CAD build for the part. Positions are in the model's coordinates, mm. A direction names the side the tool comes from. Give positions to 0.01 mm unless a question says otherwise; leave off trailing zeros. Write each loop counter-clockwise with the first axis right and the second up, starting at its lowest first coordinate (ties: lowest second). Pieces come first, ordered by that corner, then holes. Notation, with made-up numbers: (31.25, -14) -> (88.25, -14) arc R18 ccw to (88.25, 15) -> close; hole circle Ø4 at (83, -26.75). An arc over 180 degrees is marked (long way). Answer in a Markdown table with one row per item. Add a question column.
```python
from build123d import *

# Parameters (mm, degrees)
SKETCH3_W           = 800
SKETCH3_H           = 170
SKETCH3_W_2         = 740
SKETCH3_H_2         = 150
BOSS_EXTRUDE1_DEPTH = 10
BOSS_EXTRUDE2_DEPTH = 500
SKETCH5_W           = 800
SKETCH5_H           = 170
SKETCH5_W_2         = 740
SKETCH5_H_2         = 148.57875962
BOSS_EXTRUDE3_DEPTH = 10
SKETCH7_R           = 74.28937981
BOSS_EXTRUDE6_DEPTH = 500
SKETCH6_R           = 10
CUT_EXTRUDE1_DEPTH  = 521
BOSS_EXTRUDE8_DEPTH = 50
CUT_EXTRUDE2_DEPTH  = 20
SKETCH10_W          = 10.613943808
SKETCH10_H          = 30
BOSS_EXTRUDE9_DEPTH = 530


with BuildPart() as part:
    # Sketch3 → Boss-Extrude1 (new body)
    with BuildSketch(Plane.XY):
        with Locations((140, 0)):
            Rectangle(SKETCH3_W, SKETCH3_H)
        with Locations((140, 0)):
            Rectangle(SKETCH3_W_2, SKETCH3_H_2, mode=Mode.SUBTRACT)
    extrude(amount=BOSS_EXTRUDE1_DEPTH)

    # Sketch4 → Boss-Extrude2 (add)
    with BuildSketch(Plane.XY.offset(10)):
        with BuildLine():
            Line((-245, 84.28937981), (525, 84.28937981))
            ThreePointArc((525, 84.28937981), (609.28937981, 0), (525, -84.28937981))
            Line((525, -84.28937981), (-245, -84.28937981))
            ThreePointArc((-245, -84.28937981), (-329.28937981, 0), (-245, 84.28937981))
        make_face()
        with BuildLine():
            Line((-245, 74.28937981), (525, 74.28937981))
            ThreePointArc((525, 74.28937981), (599.28937981, 0), (525, -74.28937981))
            Line((525, -74.28937981), (-245, -74.28937981))
            ThreePointArc((-245, -74.28937981), (-319.28937981, 0), (-245, 74.28937981))
        make_face(mode=Mode.SUBTRACT)
    extrude(amount=BOSS_EXTRUDE2_DEPTH)

    # Sketch5 → Boss-Extrude3 (add)
    with BuildSketch(Plane.XY.offset(510)):
        with Locations((140, 0)):
            Rectangle(SKETCH5_W, SKETCH5_H)
        with Locations((140, 0)):
            Rectangle(SKETCH5_W_2, SKETCH5_H_2, mode=Mode.SUBTRACT)
    extrude(amount=BOSS_EXTRUDE3_DEPTH)

    # Sketch7 → Boss-Extrude6 (add)
    with BuildSketch(Plane.XY.offset(10)):
        with Locations((-245, 0)):
            Circle(SKETCH7_R)
        with Locations((525, 0)):
            Circle(SKETCH7_R)
    extrude(amount=BOSS_EXTRUDE6_DEPTH)

    # Sketch6 → Cut-Extrude1 (cut, through all)
    with BuildSketch(Plane.XY.offset(520)):
        with Locations((-245, 0)):
            Circle(SKETCH6_R)
        with Locations((525, 0)):
            Circle(SKETCH6_R)
    extrude(amount=-CUT_EXTRUDE1_DEPTH, mode=Mode.SUBTRACT)

    # Sketch8 → Boss-Extrude8 (add)
    with BuildSketch(Plane.XY.offset(520)):
        with BuildLine():
            Line((-245, 200), (525, 200))
            ThreePointArc((525, 200), (725, 0), (525, -200))
            Line((525, -200), (-245, -200))
            ThreePointArc((-245, -200), (-445, 0), (-245, 200))
        make_face()
    boss_extrude8 = extrude(amount=BOSS_EXTRUDE8_DEPTH)

    # Sketch9 → Cut-Extrude2 (cut)
    with BuildSketch(Plane(origin=(0, 0, 520), x_dir=(-1, 0, 0), z_dir=(0, 0, -1))):
        with BuildLine():
            Line((-525, 172.743663041), (245, 172.743663041))
            ThreePointArc((245, 172.743663041), (417.743663041, 0), (245, -172.743663041))
            Line((245, -172.743663041), (-525, -172.743663041))
            ThreePointArc((-525, -172.743663041), (-697.743663041, 0), (-525, 172.743663041))
        make_face()
        with BuildLine():
            Line((-525, -142.743663041), (245, -142.743663041))
            ThreePointArc((245, -142.743663041), (387.743663041, 0), (245, 142.743663041))
            Line((245, 142.743663041), (-525, 142.743663041))
            ThreePointArc((-525, 142.743663041), (-667.743663041, 0), (-525, -142.743663041))
        make_face(mode=Mode.SUBTRACT)
    cut_extrude2 = extrude(amount=-CUT_EXTRUDE2_DEPTH, mode=Mode.SUBTRACT)

    # Sketch10 → Boss-Extrude9 (add)
    with BuildSketch(Plane(origin=(0, 0, 540), x_dir=(-1, 0, 0), z_dir=(0, 0, -1))):
        with Locations((135.520291363, 157.743663041)):
            Rectangle(SKETCH10_W, SKETCH10_H)
        with Locations((-164.479708637, 157.743663041)):
            Rectangle(SKETCH10_W, SKETCH10_H)
        with Locations((-464.479708637, 157.743663041)):
            Rectangle(SKETCH10_W, SKETCH10_H)
    extrude(amount=BOSS_EXTRUDE9_DEPTH)

    # Mirror1: Boss-Extrude8, Cut-Extrude2 across plane
    add(boss_extrude8.mirror(Plane(origin=(0, 0, 260), x_dir=(1, 0, 0), z_dir=(0, 0, -1))))
    add(cut_extrude2.mirror(Plane(origin=(0, 0, 260), x_dir=(1, 0, 0), z_dir=(0, 0, -1))), mode=Mode.SUBTRACT)


solid = part.part
```
Item 1: Slice it at C-C, the plane y = 159. List the corners of the cut face in (x, z), then the cut area to 3 significant figures.
Item 2: Probe L1, parallel to Z at x = 508.5, y = 4.5; L2, parallel to Y at x = 10.5, z = 169; L3, parallel to Z at x = -192.5, y = 62. List the from-to ranges inside material, lowest first. Write a range as from..to.
Item 3: Which spindle directions (+Z, -Z, +X, -X, +Y, -Y) get a long thin tool onto all of the face, cutting with end or side? Do faces 1 (the face through (145, -84.289, 256)), 2 (the face through (-417.7, 3.8, 529.9)), 3 (the face through (567, 1, 510)). Say none if no direction does.
Item 4: Slice it at A-A, the plane z = 403. List the corners of the cut face in (x, y).
Item 5: Mould opens along X. For faces 4 (the face through (609.27, 1.85, 256.5)), 5 (the face through (487, 1, 10)), 6 (the face through (-286, 1, 10)), 7 (the face through (487, 1, 510)) say: released by +X, released by -X, zero draft, split by the parting line, or undercut.
Item 6: Slice it at B-B, the plane x = 571.5. List the corners of the cut face in (y, z).
Item 7: Drop flat-ended pins along their axis: pin 1 Ø2 at (x, z) = (158, 200) entering from +Y; pin 2 Ø3 at (y, z) = (6.5, 514.5) entering from +X; pin 3 Ø3 at (x, z) = (-286.5, 136.5) entering from +Y. Give the stop position or say it passes through.
Answer key:
| question | item | result |
|---|---|---|
| 1 | outline | (-366.32, -50) -> (646.32, -50) -> (646.32, 0) -> (592.52, 0) -> (592.52, -20) -> (-312.52, -20) -> (-312.52, 0) -> (-366.32, 0) -> close; (-366.32, 520) -> (-312.52, 520) -> (-312.52, 540) -> (-140.83, 540) -> (-140.83, 10) -> (-130.21, 10) -> (-130.21, 540) -> (159.17, 540) -> (159.17, 10) -> (169.79, 10) -> (169.79, 540) -> (459.17, 540) -> (459.17, 10) -> (469.79, 10) -> (469.79, 540) -> (592.52, 540) -> (592.52, 520) -> (646.32, 520) -> (646.32, 570) -> (-366.32, 570) -> close |
| 1 | area | 81,900 mm² |
| 2 | L1 | z = -50..0, 10..510, 520..570 |
| 2 | L2 | y = -84.29..-74.29, 74.29..84.29 |
| 2 | L3 | z = -50..0, 520..570 |
| 3 | face 1 | +X, -X, -Y |
| 3 | face 2 | none |
| 3 | face 3 | +X, +Y, -Y |
| 4 | outline | (-245, -84.29) -> (525, -84.29) arc R84.29 ccw to (525, 84.29) -> (-245, 84.29) arc R84.29 ccw to start; (-140.83, 142.74) -> (-130.21, 142.74) -> (-130.21, 172.74) -> (-140.83, 172.74) -> close; (159.17, 142.74) -> (169.79, 142.74) -> (169.79, 172.74) -> (159.17, 172.74) -> close; (459.17, 142.74) -> (469.79, 142.74) -> (469.79, 172.74) -> (459.17, 172.74) -> close; hole circle Ø20 at (-245, 0); hole (-245, -74.29) -> (525, -74.29) arc R74.29 cw to (525, 74.29) -> (-245, 74.29) arc R74.29 cw to start; hole circle Ø20 at (525, 0) |
| 5 | face 4 | released by +X |
| 5 | face 5 | undercut |
| 5 | face 6 | zero draft |
| 5 | face 7 | undercut |
| 6 | outline | (-194.52, -50) -> (194.52, -50) -> (194.52, 0) -> (166.37, 0) -> (166.37, -20) -> (134.96, -20) -> (134.96, 0) -> (-134.96, 0) -> (-134.96, -20) -> (-166.37, -20) -> (-166.37, 0) -> (-194.52, 0) -> close; (-194.52, 520) -> (-166.37, 520) -> (-166.37, 540) -> (-134.96, 540) -> (-134.96, 520) -> (134.96, 520) -> (134.96, 540) -> (166.37, 540) -> (166.37, 520) -> (194.52, 520) -> (194.52, 570) -> (-194.52, 570) -> close; (-70.3, 10) -> (70.3, 10) -> (70.3, 510) -> (-70.3, 510) -> close |
| 7 | pin 1 | stops at y = 84.29 |
| 7 | pin 2 | stops at x = 540 |
| 7 | pin 3 | stops at y = 74.19 |
